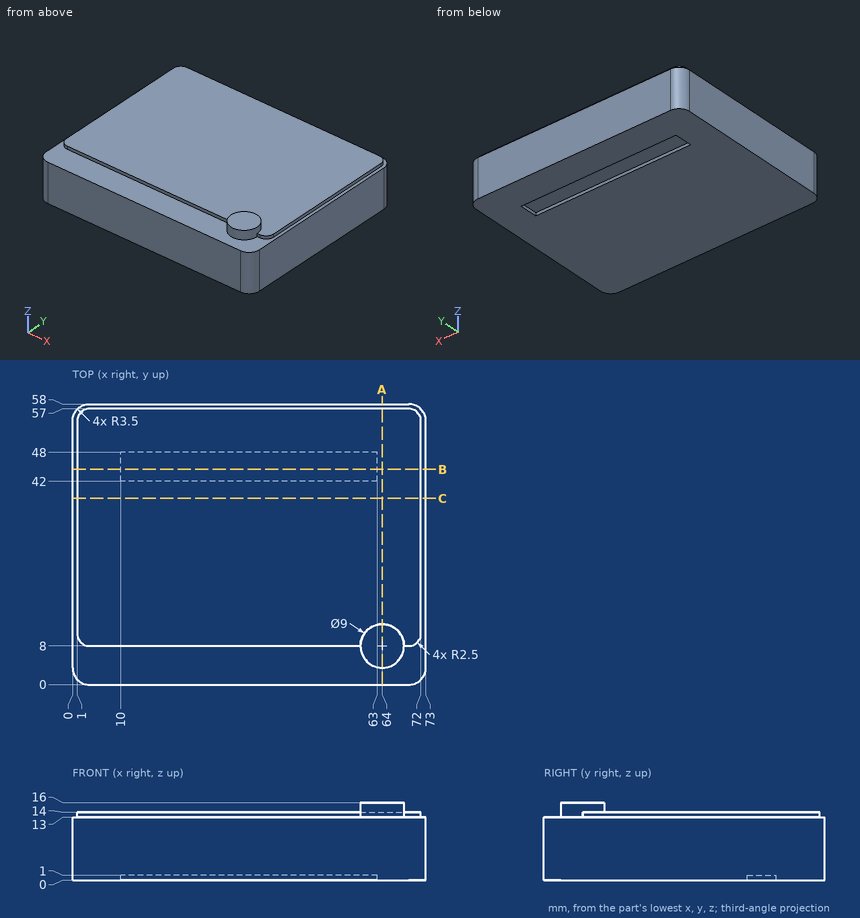
Can you work these out from the drawing? Everything is in mm from the part's minimum corner. Coordinates: 2 decimals unless noted, no trailing zeros. Write each loop counter-clockwise with the first axis right and the second up, starting at its lowest first coordinate (ties: lowest second). Pieces come first, ordered by that corner, then holes. Notation, with made-up numbers: (36.25, 25) -> (57.25, 25) arc R32 ccw to (57.25, 54) -> close; hole circle Ø3 at (86.5, 37). An arc over 180 degrees is marked (long way). Return JSON: item names as keys, results as strings.
(1) I'm going to push flat-ended pins straight in: pin 1 (24.5 mm diameter, centred on x = 23.5, y = 36, fed in from +Z); pin 2 (0.8 mm diameter, centred on x = 27, z = 13.5, fed in from +Y); pin 3 (0.5 mm diameter, centred on x = 31.5, z = 13.5, fed in from -Y). Where does each tip first touch, or does it pass through?
Numbers:
{"pin 1": "stops at z = 14", "pin 2": "stops at y = 57", "pin 3": "stops at y = 8"}
(2) I need wall thicknesses on L1, parallel to Z at x = 49, y = 5.5; L2, parallel to Z at x = 67, y = 45; L3, parallel to X at y = 31, z = 13.75. Which ranges of each line are inside material? Lowest first, please.
Numbers:
{"L1": "z = 0 to 13", "L2": "z = 0 to 14", "L3": "x = 1 to 72"}
(3) Imagine slicing it at A-A, the plane x = 64. Please give me the cut outline in (y, z).
Numbers:
{"outline": "(0, 0) -> (58, 0) -> (58, 13) -> (57, 13) -> (57, 14) -> (12.5, 14) -> (12.5, 16) -> (3.5, 16) -> (3.5, 13) -> (0, 13) -> close"}
(4) Imagine slicing it at B-B, the plane y = 44.5. Please give me the cut outline in (x, z), then the cut area to 3 significant figures.
Numbers:
{"outline": "(0, 0) -> (10, 0) -> (10, 1) -> (63, 1) -> (63, 0) -> (73, 0) -> (73, 13) -> (72, 13) -> (72, 14) -> (1, 14) -> (1, 13) -> (0, 13) -> close", "area": "967 mm2"}
(5) Imagine slicing it at C-C, the plane y = 38.5. Please give me the cut outline in (x, z), then the cut area to 3 significant figures.
Numbers:
{"outline": "(0, 0) -> (73, 0) -> (73, 13) -> (72, 13) -> (72, 14) -> (1, 14) -> (1, 13) -> (0, 13) -> close", "area": "1,020 mm2"}
